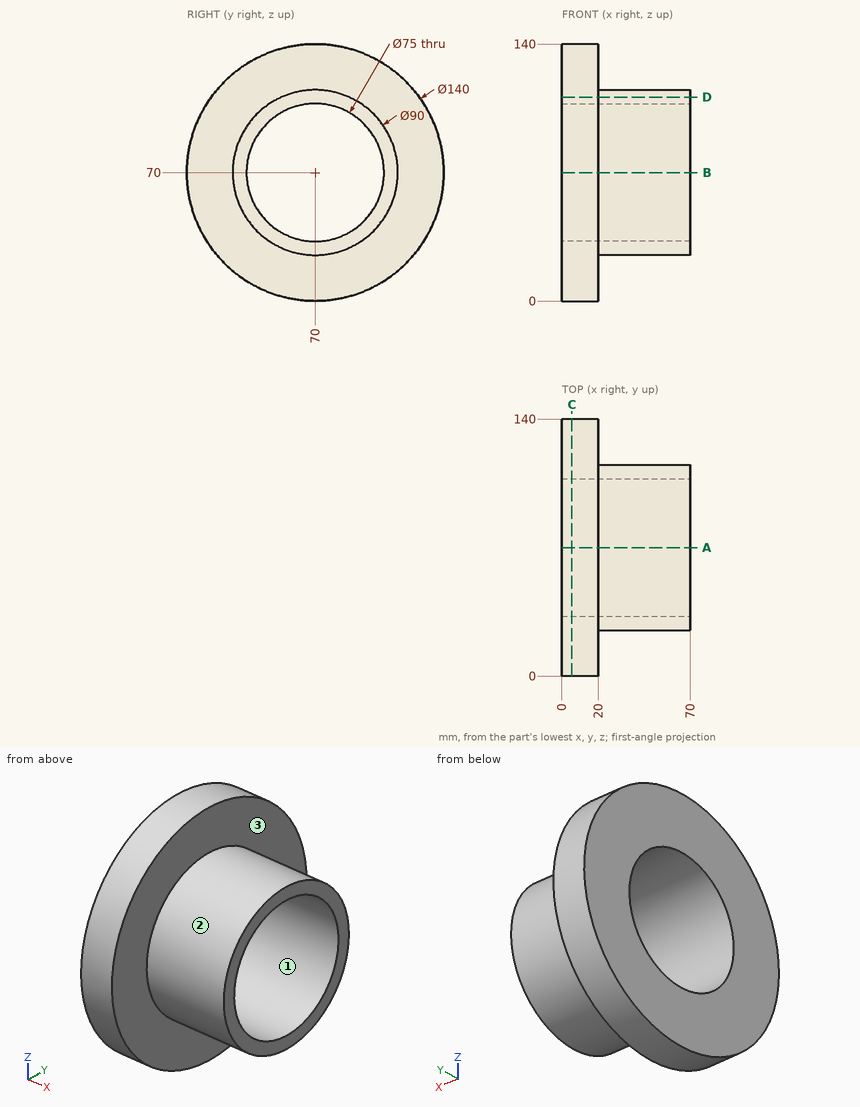
For this review, use the dimensioned drawing (mm, ordinates from the lowest corner) and the shaded views. Round coordinates to 2 decimals unless told otherwise and drop trailing zeros. Write each loop counter-clockwise with the first axis right and the second up, starting at its lowest first coordinate (ties: lowest second). Pieces come first, ordered by that corner, then holes. Notation, with made-up numbers: (63, 28) - (102, 28) arc R9 ccw to (102, 32) - close; hole circle Ø1 at (7, -8). An arc over 180 degrees is marked (long way). Use CSV: the item, a comma, the result in double quotes.
1) Wall thickness on line 1 along Y through (x, z) = (39, 70); line 2 along X through (y, z) = (45.5, 129.5); line 3 along Y through (x, z) = (46.5, 61): over which ranges is each line inside the solid? List them lowest first. Write a range as from..to.
Conclusion:
line 1,"y = 25..32.5, 107.5..115"
line 2,"x = 0..20"
line 3,"y = 25.91..33.6, 106.4..114.09"
2) Add section D-D on z = 111. Write out the cut boundary in (x, y), and give its area (3 significant figures).
Conclusion:
outline,"(0, 13.26) - (20, 13.26) - (20, 51.45) - (70, 51.45) - (70, 88.55) - (20, 88.55) - (20, 126.74) - (0, 126.74) - close"
area,"4,120 mm^2"
3) Add section A-A on y = 70. Write out the cut boundary in (x, z).
Conclusion:
outline,"(0, 0) - (20, 0) - (20, 25) - (70, 25) - (70, 32.5) - (0, 32.5) - close; (0, 107.5) - (70, 107.5) - (70, 115) - (20, 115) - (20, 140) - (0, 140) - close"
4) Add section C-C on x = 5.5. Write out the cut boundary in (y, z), and give its area (3 significant figures).
Conclusion:
outline,"circle Ø140 at (70, 70); hole circle Ø75 at (70, 70)"
area,"11,000 mm^2"
5) The part is to be moulded in two halves that separate along Z. For the marked faces 1, 2 and 3, say which applies: pulls with the +Z half, pulls with the -Z half, needs draft (parallel to the pull), parting line crosses it, or undercut.
Conclusion:
face 1,"undercut"
face 2,"parting line crosses it"
face 3,"needs draft"
6) Clearance check with flat-ended pins moving along their axes: pin 1 Ø6 at (x, z) = (31.5, 96) entering from -Y; pin 2 Ø6 at (x, y) = (40.5, 98) entering from -Z; pin 3 Ø6 at (x, y) = (57.5, 21.5) entering from -Z; pin 4 Ø12 at (x, y) = (18, 25) entering from -Z. State where each tip first meets the part, or that it passes through.
Conclusion:
pin 1,"stops at y = 31.32"
pin 2,"stops at z = 32.58"
pin 3,"passes through"
pin 4,"stops at z = 11.87"
